Geometry check sheet. Reference: the model listing, model coordinates, mm. A direction names the side the tool comes from. Round coordinates to 2 decimals unless told otherwise and drop trailing zeros. Write each loop counter-clockwise with the first axis right and the second up, starting at its lowest first coordinate (ties: lowest second). Pieces come first, ordered by that corner, then holes. Notation, with made-up numbers: M -37.75,4 L 13.25,4 A14 cw 13.25,27 Z; hole C 1.5,-14 d5. An arc over 180 degrees is marked long. One line per item, written item: value. Start each with the question number.
1. Access from +Z, -Z, +X, -X, +Y, -Y to the whole of each face (thin tool, end or side, straight path). Record for faces 4 (the flat face through (42, 0, 5)), 5 (the flat face through (19, -12, 6.1)), 6 (the cylindrical face through (49.4, 22.43, 6.06)).
2. Scan lines: probe 1 along X at (y, z) = (2, 2.75); probe 2 along X at (y, z) = (12, 6.25); probe 3 along X at (y, z) = (-11.5, 7.5). Record each from-to range of solid material in increasing order. Write a range as [from, to].
3. Section check B-B (x = -19). Record the boundary of the cut face in (y, z), and give its area (3 significant figures).
4. Depth check by flat-ended pin: P1, Ø5, axis at x = 18, y = 14.085, coming from the +Z side; P2, Ø2.5, axis at x = -18.5, y = 14.085, coming from the -Z side. Enter the tip coordinate at first touch or a pass-through.
5. Release check for a two-part mould opening along Y. For faces 1 (the flat face through (-1, 0, 10)), 2 (the cylindrical face through (-16.55, 14.17, 3.01)), 3 (the cylindrical face through (0.67, 22.43, 0.6)) record: pulls with the +Y half, pulls with the -Y half, needs draft (parallel to the pull), parting line crosses it, or undercut.
6. Section check D-D (z = 9). Record the boundary of the cut face in (x, y) (3 decimals), and give its area (3 significant figures).
7. Section check C-C (z = 4). Record the boundary of the cut face in (x, y) (3 decimals).
8. Section check A-A (x = -36.5). Record the boundary of the cut face in (y, z).
from build123d import *

# Parameters (mm, degrees)
SKETCH_W         = 100
SKETCH_H         = 46
PAD_DEPTH        = 10
HOLE_D           = 3.9
HOLE_CBORE_D     = 8
HOLE_CBORE_DEPTH = 3.9
FILLET_R         = 2
FILLET001_R      = 2
FILLET002_R      = 2
FILLET003_R      = 2


with BuildPart() as part:
    # Sketch → Pad (new body)
    with BuildSketch(Plane.XY):
        Rectangle(SKETCH_W, SKETCH_H)
        with BuildLine():
            ThreePointArc((42, 11.5), (38.5, 15), (35, 11.5))
            Line((35, 11.5), (35, -11.5))
            ThreePointArc((35, -11.5), (38.5, -15), (42, -11.5))
            Line((42, -11.5), (42, 11.5))
        make_face(mode=Mode.SUBTRACT)
        with BuildLine():
            ThreePointArc((-33, 11.5), (-36.5, 15), (-40, 11.5))
            Line((-40, 11.5), (-40, -11.5))
            ThreePointArc((-40, -11.5), (-36.5, -15), (-33, -11.5))
            Line((-33, -11.5), (-33, 11.5))
        make_face(mode=Mode.SUBTRACT)
    extrude(amount=PAD_DEPTH)

    # Hole (through all)
    with Locations(Plane.XY.offset(10)):
        with Locations((-18.5, 14.085), (18, 14.085), (-18, -13.585), (18.5, -14.085)):
            CounterBoreHole(HOLE_D / 2, HOLE_CBORE_D / 2, HOLE_CBORE_DEPTH)

    # Fillet
    fillet_edges = [part.edges().sort_by_distance(p)[0] for p in [
        (-50, 0, 0),
    ]]
    fillet(fillet_edges, radius=FILLET_R)

    # Fillet001
    fillet001_edges = [part.edges().sort_by_distance(p)[0] for p in [
        (1, 23, 0),
    ]]
    fillet(fillet001_edges, radius=FILLET001_R)

    # Fillet002
    fillet002_edges = [part.edges().sort_by_distance(p)[0] for p in [
        (50, -1, 0),
    ]]
    fillet(fillet002_edges, radius=FILLET002_R)

    # Fillet003
    fillet003_edges = [part.edges().sort_by_distance(p)[0] for p in [
        (0, -23, 0),
    ]]
    fillet(fillet003_edges, radius=FILLET003_R)


solid = part.part
Result sheet:
1. face 4: +Z, -Z
1. face 5: +Z
1. face 6: +Z, -Z, +X, +Y
2. probe 1: x = [-50, -40], [-33, 35], [42, 50]
2. probe 2: x = [-50, -39.96], [-33.04, -21.91], [-15.09, 14.59], [21.41, 35.04], [41.96, 50]
2. probe 3: x = [-50, -40], [-33, -21.41], [-14.59, 15.45], [21.55, 35], [42, 50]
3. outline: M -23,2 A2 ccw -21,0 L -15.26,0 L -15.26,6.1 L -17.46,6.1 L -17.46,10 L -23,10 Z; M -11.91,0 L 12.2,0 L 12.2,6.1 L 10.12,6.1 L 10.12,10 L -9.71,10 L -9.71,6.1 L -11.91,6.1 Z; M 15.97,0 L 21,0 A2 ccw 23,2 L 23,10 L 18.05,10 L 18.05,6.1 L 15.97,6.1 Z
3. area: 354 mm2
4. P1: stops at z = 6.1
4. P2: passes through
5. face 1: needs draft
5. face 2: undercut
5. face 3: pulls with the +Y half
6. outline: M -50,-21 A2 ccw -48,-23 L 48,-23 A2 ccw 50,-21 L 50,21 A2 ccw 48,23 L -48,23 A2 ccw -50,21 Z; hole M -40,-11.5 A3.5 ccw -33,-11.5 L -33,11.5 A3.5 ccw -40,11.5 Z; hole C -18.5,14.085 d8; hole C -18,-13.585 d8; hole C 18,14.085 d8; hole C 18.5,-14.085 d8; hole M 35,-11.5 A3.5 ccw 42,-11.5 L 42,11.5 A3.5 ccw 35,11.5 Z
6. area: 4,000 mm2
7. outline: M -50,-21 A2 ccw -48,-23 L 48,-23 A2 ccw 50,-21 L 50,21 A2 ccw 48,23 L -48,23 A2 ccw -50,21 Z; hole M -40,-11.5 A3.5 ccw -33,-11.5 L -33,11.5 A3.5 ccw -40,11.5 Z; hole C -18.5,14.085 d3.9; hole C -18,-13.585 d3.9; hole C 18,14.085 d3.9; hole C 18.5,-14.085 d3.9; hole M 35,-11.5 A3.5 ccw 42,-11.5 L 42,11.5 A3.5 ccw 35,11.5 Z
8. outline: M -23,2 A2 ccw -21,0 L -15,0 L -15,10 L -23,10 Z; M 15,0 L 21,0 A2 ccw 23,2 L 23,10 L 15,10 Z
